Model file for the job. Use its own axes, mm. A direction names the side the tool comes from. Round coordinates to 2 decimals unless told otherwise and drop trailing zeros. Order: outer loops, then holes, each group sorted by start corner. A loop starts at its lowest first (then second) coordinate and runs counter-clockwise, first axis right, second up. Notation, with made-up numbers: (23.25, 71) - (45.25, 71) arc R29 cw to (45.25, 95) - close; hole circle Ø9 at (-4, 67.5). An arc over 180 degrees is marked (long way). Answer as CSV lines item,"result". Start each with the question number.
1. Band-saw the part on D-D on y = -74. List the corners of the cut face in (x, z), then the cut area to 3 significant figures.
2. Pull direction Y, two halves, no side cores. Call faces 1 (the face through (2, 53, 38)), 2 (the face through (10, 92.5, 20)), 3 (the face through (4, -40, 15)), 4 (the face through (8.056, 78.837, 19.86)): released by +Y, released by -Y, zero draft, split by the parting line, or undercut.
3. Band-saw the part on C-C on z = 22. List the corners of the cut face in (x, y), then the cut area to 3 significant figures.
4. Wall check: line 1 along Z through (x, y) = (2.35, 25); line 2 along X through (y, z) = (-59, 23.5); line 3 along Z through (x, y) = (1, -4). Give the ranges that are in metal, low to high. Write a range as [from, to].
5. Pin check, flat tips, straight feed: pin 1 Ø19 at (y, z) = (9, 24.5) entering from +X; pin 2 Ø8 at (y, z) = (87, 16.5) entering from -X; pin 3 Ø6 at (x, y) = (9, 80.5) entering from +Z; pin 4 Ø5 at (x, y) = (7, -7) entering from -Z (3 decimals). Stop position of each tip, or through.
6. Band-saw the part on A-A on z = 4. List the corners of the cut face in (x, y).
7. 3-axis set-ups, long thin cutter, end or side, ignore diameter. For faces 5 (the face through (4, 74, 10)), 6 (the face through (8, 83, 30)), 7 (the face through (4, 22, 19)): which of +Z, -Z, +X, -X, +Y, -Y reach the whole face in a straight line?
8. Band-saw the part on B-B on y = -25. List the corners of the cut face in (x, z).
Solid Edge part; units mm, degrees
sketch "Sketch1" plane through (0, 0, 0) normal (0, 0, 1) x (1, 0, 0)
  line L0 (0, 72.5) -> (8, 85)
  line L1 (8, 85) -> (12, 85)
  line L2 (12, 85) -> (4, 72.5)
  line L3 (4, 72.5) -> (4, -30)
  line L4 (4, -30) -> (12, -50)
  line L5 (12, -50) -> (12, -92)
  line L6 (12, -92) -> (8, -92)
  line L7 (8, -92) -> (8, -50)
  line L8 (8, -50) -> (0, -30)
  line L9 (0, -30) -> (0, 72.5)
  dimension "D1" = 12
  dimension "D2" = 8
  dimension "D3" = 8
  dimension "D4" = 8
extrude "Protrusion1" add sketch "Sketch1" along normal blind 30
hole "Hole1" at (0, 25, 4) direction (1, 0, 0) diameter 3.4 end up to next start chamfer 0.3 start chamfer angle 45 end chamfer 0.3 end chamfer angle 45
hole "Hole2" at (0, -25, 4) direction (1, 0, 0) diameter 3.4 end up to next start chamfer 0.3 start chamfer angle 45 end chamfer 0.3 end chamfer angle 45
sketch "Sketch2" plane through (0, 0, 0) normal (1, 0, 0) x (0, 1, 0)
  line L0 (47.5, 0) -> (55, 10)
  line L1 (55, 10) -> (85, 10)
  line L2 (85, 10) -> (85, 0)
  line L3 (85, 0) -> (47.5, 0)
  dimension "D1" = 85
  dimension "D2" = 85
  dimension "D3" = 55
extrude "front_bearing_cutout" cut sketch "Sketch2" along normal blind 46.5167
sketch "Sketch3" plane through (8, -71, 15) normal (-1, 0, 0) x (0, -1, 0)
  line L0 (-19, -15) -> (-9, -5)
  line L1 (-9, -5) -> (21, -5)
  line L2 (21, -5) -> (21, -15)
  line L3 (21, -15) -> (-19, -15)
  dimension "D1" = 21
  dimension "D2" = 21
  dimension "D3" = 9
extrude "Cutout1" cut sketch "Sketch3" against normal up to next
sketch "Sketch4" plane through (6, -2.25, 30) normal (0, 0, 1) x (0, -1, 0)
  line L0 (-87.25, 6) -> (-87.25, 2)
  line L1 (-87.25, 2) -> (-94.75, 2)
  line L2 (-94.75, 2) -> (-94.75, 6)
  line L3 (-94.75, 6) -> (-87.25, 6)
  dimension "D1" = 94.75
extrude "Protrusion2" add sketch "Sketch4" against normal up to vertex (20 mm away)
sketch "Sketch5" plane through (0, 21.25, 15) normal (-1, 0, 0) x (0, -1, 0)
  line L0 (-51.25, 15) -> (-43.25, 23)
  line L1 (-43.25, 23) -> (-19.25, 23)
  line L2 (-11.25, 15) -> (-19.25, 23)
  line L3 (-51.25, 15) -> (-11.25, 15)
  dimension "D1" = 11.25
  dimension "D2" = 51.25
  dimension "D3" = 43.25
extrude "Protrusion3" add sketch "Sketch5" against normal up to vertex (4 mm away)
properties material "Polyethylene, low density"
Reply:
1,outline,"(8, 10) - (12, 10) - (12, 30) - (8, 30) - close"
1,area,"80.0 mm2"
2,face 1,"zero draft"
2,face 2,"released by +Y"
2,face 3,"released by -Y"
2,face 4,"undercut"
3,outline,"(0, -30) - (8, -50) - (8, -92) - (12, -92) - (12, -50) - (4, -30) - (4, 72.5) - (12, 85) - (12, 92.5) - (8, 92.5) - (8, 85) - (0, 72.5) - close"
3,area,"738 mm2"
4,line 1,"z = [0, 2.3], [5.7, 30]"
4,line 2,"x = [8, 12]"
4,line 3,"z = [0, 30]"
5,pin 1,"stops at x = 4"
5,pin 2,"stops at x = 6.72"
5,pin 3,"stops at z = 30"
5,pin 4,"passes through"
6,outline,"(0, -30) - (8, -50) - (8, -56) - (12, -56) - (12, -50) - (4, -30) - (4, -27) - (3.7, -26.7) - (0.3, -26.7) - (0, -27) - close; (0, -23) - (0.3, -23.3) - (3.7, -23.3) - (4, -23) - (4, 23) - (3.7, 23.3) - (0.3, 23.3) - (0, 23) - close; (0, 27) - (0.3, 26.7) - (3.7, 26.7) - (4, 27) - (4, 50.5) - (0, 50.5) - close"
7,face 5,"-Z, +X, -X, +Y"
7,face 6,"+Z, +X, -X, +Y"
7,face 7,"+Z, -Z, +X"
8,outline,"(0, 0) - (4, 0) - (4, 2) - (3.7, 2.3) - (0.3, 2.3) - (0, 2) - close; (0, 6) - (0.3, 5.7) - (3.7, 5.7) - (4, 6) - (4, 30) - (0, 30) - close"
